Check sheet for the modelled part. Datum: model origin and axes. Units: mm. Face numbers are marked on the shaded views. A direction names the side the tool comes from. Give positions to 0.01 mm unless a question says otherwise; leave off trailing zeros. Loops run counter-clockwise (first coordinate to the right, second up) from the corner with the lowest first, then second, coordinate; pieces in that order, holes last. Notation, with made-up numbers: (89, 53) - (122, 53) arc R34 ccw to (122, 92) - close; hole circle Ø3 at (77, -25.75). An arc over 180 degrees is marked (long way). Use CSV: the item, a comma, the result in double quotes.
Autodesk Inventor part; units mm, degrees
ref_plane "YZ Plane" through (0, 0, 0) normal (1, 0, 0) x (0, 1, 0)
ref_plane "XZ Plane" through (0, 0, 0) normal (0, 1, 0) x (-1, 0, 0)
ref_plane "XY Plane" through (0, 0, 0) normal (0, 0, 1) x (1, 0, 0)
sketch "Sketch1" plane through (0, 0, 0) normal (0, 0, 1) x (1, 0, 0)
  line L0 (-62.4, 25.45) -> (62.4, 25.45)
  line L1 (62.4, 25.45) -> (62.4, -25.45)
  line L2 (62.4, -25.45) -> (-62.4, -25.45)
  line L3 (-62.4, -25.45) -> (-62.4, 25.45)
  point P0 (0, 0)
  dimension "d0" = 124.8
  dimension "d1" = 50.9
  dimension "d2" = 62.4
  dimension "d3" = 25.45
extrude "Extrusion1" add sketch "Sketch1" along normal blind 10.0076
fillet "Fillet1" radius 3.175 3 edges at (62.4, 25.45, 5.0038) (62.4, -25.45, 5.0038) (-62.4, -25.45, 5.0038)
fillet "Fillet2" radius 3.175 1 edges at (-62.4, 25.45, 5.0038)
sketch "Sketch5" plane through (0, 0, 10.0076) normal (0, 0, 1) x (1, 0, 0)
  line L0 (-8.885, 4.137) -> (9.115, 4.137)
  line L1 (9.115, 4.137) -> (9.115, 16.687)
  line L2 (9.115, 16.687) -> (-8.885, 16.687)
  line L3 (-8.885, 16.687) -> (-8.885, 4.137)
  circle A0 centre (-12.38, 10.412) radius 1.7859
  circle A1 centre (12.61, 10.412) radius 1.7859
  circle A2 centre (26.495, 9.117) radius 6.731
  line L4 (2.175, 8.737) -> (14.175, 8.737)
  line L5 (14.175, 8.737) -> (14.175, 16.737)
  line L6 (14.175, 16.737) -> (2.175, 16.737)
  line L7 (2.175, 16.737) -> (2.175, 8.737)
  line L8 (2.175, 13.737) -> (2.175, 8.737)
  line L9 (2.175, 8.737) -> (14.175, 8.737)
  line L10 (14.175, 8.737) -> (14.175, 13.737)
  line L11 (14.175, 13.737) -> (2.175, 13.737)
  line L12 (47.045, 8.237) -> (63.045, 8.237)
  line L13 (63.045, 8.237) -> (63.045, 16.737)
  line L14 (63.045, 16.737) -> (47.045, 16.737)
  line L15 (47.045, 16.737) -> (47.045, 8.237)
  arc A3 (-8.885, 7.412) -> (-6.885, 5.412) centre (-6.885, 7.412) ccw
  line L16 (-8.885, 13.412) -> (-8.885, 7.412)
  arc A4 (-6.885, 15.412) -> (-8.885, 13.412) centre (-6.885, 13.412) ccw
  line L17 (7.115, 15.412) -> (-6.885, 15.412)
  arc A5 (9.115, 13.412) -> (7.115, 15.412) centre (7.115, 13.412) ccw
  line L18 (9.115, 7.412) -> (9.115, 13.412)
  arc A6 (7.115, 5.412) -> (9.115, 7.412) centre (7.115, 7.412) ccw
  line L19 (-6.885, 5.412) -> (7.115, 5.412)
  point P0 (0, 0)
extrude "Extrusion5" cut sketch "Sketch5" against normal up to surface (10.0076 mm away) contours L3 A4 L17 L7 L4 L1 A6 L19 A3 | L4 L7 L11 A5 L1 | L4 A1 | A1 L5 L4 | L17 A5 L11 L7 | A1 L5 | A0 picked at (13.0769, 10.2632)
properties part number "back cover"
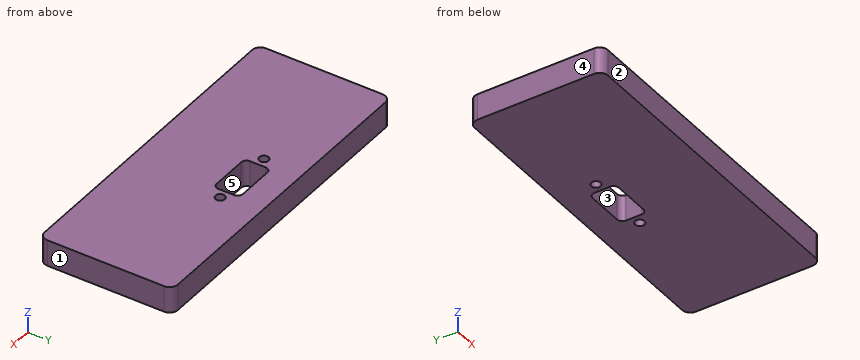
1. Scan lines: line 1 along Y through (x, z) = (12.61, 7); line 2 along Y through (x, z) = (2, 5); line 3 along X through (y, z) = (13, 9.25) (3 decimals). Record each from-to range of solid material in increasing order.
Completed:
line 1,"y = -25.45 to 8.63, 12.2 to 25.45"
line 2,"y = -25.45 to 5.41, 15.41 to 25.45"
line 3,"x = -62.4 to -8.885, 9.115 to 62.4"
2. Sectioned sample at A-A, the plane x = -12.38. Record the boundary of the cut face in (y, z), and give its area (3 significant figures).
Completed:
outline,"(-25.45, 0) - (8.63, 0) - (8.63, 10.01) - (-25.45, 10.01) - close; (12.2, 0) - (25.45, 0) - (25.45, 10.01) - (12.2, 10.01) - close"
area,"474 mm²"
3. Go/stop test with a flat-tipped pin: pin 1 Ø3 at (x, y) = (-12.38, 10.412) entering from -Z. Record where the tip stops, or that it passes through.
Completed:
pin 1,"passes through"
4. Sectioned sample at B-B, the plane z = 8.5. Record the boundary of the cut face in (x, y) (3 decimals).
Completed:
outline,"(-62.4, -22.275) arc R3.175 ccw to (-59.225, -25.45) - (59.225, -25.45) arc R3.175 ccw to (62.4, -22.275) - (62.4, 22.275) arc R3.175 ccw to (59.225, 25.45) - (-59.225, 25.45) arc R3.175 ccw to (-62.4, 22.275) - close; hole circle Ø3.572 at (-12.38, 10.412); hole (-8.885, 7.412) arc R2 ccw to (-6.885, 5.412) - (7.115, 5.412) arc R2 ccw to (9.115, 7.412) - (9.115, 13.412) arc R2 ccw to (7.115, 15.412) - (-6.885, 15.412) arc R2 ccw to (-8.885, 13.412) - close; hole circle Ø3.572 at (12.61, 10.412)"
5. Set-up check for the marked faces 4 and 5: record each of +Z, -Z, +X, -X, +Y, -Y from which the full face is reachable in a straight line by a thin tool's end or side.
Completed:
face 4,"+Z, -Z, -X, +Y, -Y"
face 5,"+Z, -Z"
6. Release check for a two-part mould opening along Y. For the marked faces 1, 2 and 3 record: released by +Y, released by -Y, zero draft, split by the parting line, or undercut.
Completed:
face 1,"zero draft"
face 2,"released by -Y"
face 3,"undercut"
